The figure shows three views and two pictorial views of one solid part (mm, origin at its lowest corner). Answer the questions. A direction names the side the tool comes from. Round coordinates to 2 decimals unless told otherwise and drop trailing zeros. Write each loop counter-clockwise with the first axis right and the second up, starting at its lowest first coordinate (ties: lowest second). Pieces come first, ordered by that corner, then holes. Notation, with made-up numbers: M -15.5,57 L 3.5,57 A23 ccw 3.5,86 Z; hole C 67.5,-25.75 d4. An arc over 180 degrees is marked long. One line per item, written item: value. Start each with the question number.
Q1. Find section A-A (x = 29). Write down the section's boundary in (y, z).
Q2. Consider probe 1 along X at (y, z) = (38.5, 1.25); probe 2 along X at (y, z) = (20, 0.45); probe 3 along Y at (x, z) = (18.5, 4.95). Determine where each line is inside the solid, lowest interval first.
Q3. Find section C-C (z = 4.45). Write down the section's boundary in (x, y).
Q4. The mould has two halves that part along Y. Classify the marked faces 3, 4, 5 and 6: released by +Y, released by -Y, zero draft, split by the parting line, or undercut.
Q5. Given pin 1 Ø2.5 at (y, z) = (52.5, 2) entering from -X; pin 2 Ø1.6 at (x, z) = (53, 4) entering from -Y; pin 3 Ø1.6 at (x, z) = (52.5, 2.5) entering from +Y, each flat-ended and moving along its own axis, determine where each tip first touches the part or whether it passes through.
Q6. A tool of negligible diameter and unlimited length cuts with its end or side. For the marked faces 1 and 2, from which of +Z, -Z, +X, -X, +Y, -Y can it reach the whole face along a straight path? Write none if from no direction.
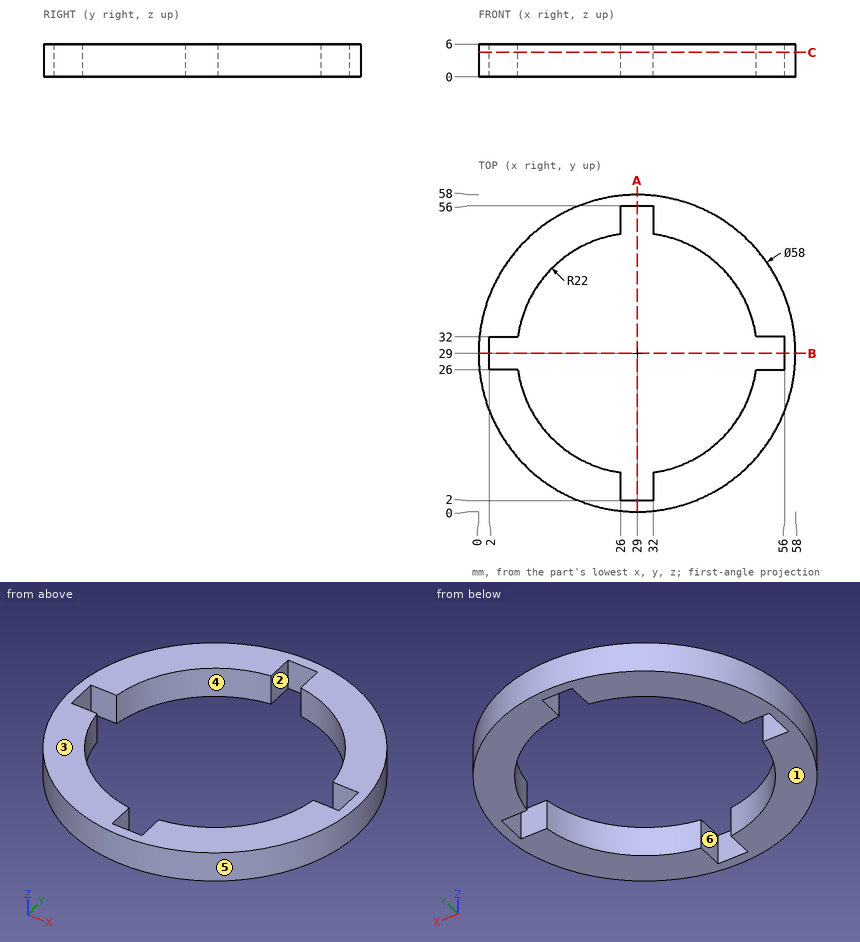
The answers:
1. outline: M 0,0 L 2,0 L 2,6 L 0,6 Z; M 56,0 L 58,0 L 58,6 L 56,6 Z
2. probe 1: 1.6 to 9.16, 48.84 to 56.4
2. probe 2: 1.43 to 8.93, 49.07 to 56.57
2. probe 3: 1.97 to 9.67, 48.33 to 56.03
3. outline: C 29,29 d58; hole M 2,26 L 7.21,26 A22 ccw 26,7.21 L 26,2 L 32,2 L 32,7.21 A22 ccw 50.79,26 L 56,26 L 56,32 L 50.79,32 A22 ccw 32,50.79 L 32,56 L 26,56 L 26,50.79 A22 ccw 7.21,32 L 2,32 Z
4. face 3: zero draft
4. face 4: undercut
4. face 5: split by the parting line
4. face 6: undercut
5. pin 1: x = 10.4
5. pin 2: y = 11.6
5. pin 3: y = 47.05
6. face 1: -Z, +X, -X, +Y, -Y
6. face 2: +Z, -Z
